Design review of the part built by this model. Coordinates are the model's own, in mm. A direction names the side the tool comes from. Give positions to 0.01 mm unless a question says otherwise; leave off trailing zeros. Write each loop counter-clockwise with the first axis right and the second up, starting at its lowest first coordinate (ties: lowest second). Pieces come first, ordered by that corner, then holes. Notation, with made-up numbers: (37.25, -15.75) -> (56.25, -15.75) arc R21 ccw to (56.25, 16.25) -> close; hole circle Ø8 at (-7.75, 14). An arc over 180 degrees is marked (long way). Answer as a JSON object with one key per item and string values.
Solid Edge part; units mm, degrees
sketch "Sketch1" plane through (0, 0, 0) normal (0, 0, 1) x (1, 0, 0)
  arc A0 (-42.2727, 39.6197) -> (-53.3598, 0) centre (-0.8768, 6.6744) ccw
  arc A1 (-53.3598, 0) -> (-25.9191, -47.548) centre (0.1673, -0.8009) ccw
  line L0 (-26.65, -48.8578) -> (-25.9191, -47.548)
  arc A2 (-54.8611, -0.0838) -> (-26.65, -48.8578) centre (0.1673, -0.8009) ccw
  arc A3 (-43.4475, 40.5523) -> (-54.8611, -0.0838) centre (-0.8768, 6.6744) ccw
  arc A4 (-9.2588, 61.3508) -> (-43.4475, 40.5523) centre (1.7356, 4.7791) ccw
  line L1 (-9.2588, 69.5332) -> (-9.2588, 61.3508)
  line L2 (5.3113, 69.5332) -> (-9.2588, 69.5332)
  line L3 (5.7406, 61.9223) -> (5.3113, 69.5332)
  arc A5 (43.4475, 40.5523) -> (5.7406, 61.9223) centre (-1.7356, 4.7791) ccw
  arc A6 (54.8611, -0.0838) -> (43.4475, 40.5523) centre (0.8768, 6.6744) ccw
  arc A7 (28.0706, -48.0371) -> (54.8611, -0.0838) centre (-0.1673, -0.8009) ccw
  line L4 (27.3009, -46.7496) -> (28.0706, -48.0371)
  arc A8 (53.3598, 0) -> (27.3009, -46.7496) centre (-0.1673, -0.8009) cw
  arc A9 (42.2727, 39.6197) -> (53.3598, 0) centre (0.8768, 6.6744) cw
  arc A10 (4.3138, 60.5824) -> (42.2727, 39.6197) centre (-1.7356, 4.7791) cw
  line L5 (3.8935, 68.0332) -> (4.3138, 60.5824)
  line L6 (-7.7588, 68.0332) -> (3.8935, 68.0332)
  line L7 (-7.7588, 68.0332) -> (-7.7588, 60.1005)
  arc A11 (-7.7588, 60.1005) -> (-42.2727, 39.6197) centre (1.7356, 4.7791) ccw
extrude "Protrusion1" add sketch "Sketch1" along normal blind 10
sketch "Sketch2" plane through (0, 10.3377, 10) normal (0, 0, 1) x (0, -1, 0)
  line L0 (8.4418, -53.9965) -> (8.4418, 54.1624)
  line L1 (8.4418, 54.1624) -> (10.3377, 53.3598)
  line L2 (10.3377, 53.3598) -> (10.3377, -53.3598)
  line L3 (10.3377, -53.3598) -> (8.4418, -53.9965)
extrude "ExtrudedProtrusion_2" add sketch "Sketch2" against normal blind 2
sketch "Sketch3" plane through (0, 10.3377, 10) normal (0, 0, 1) x (0, -1, 0)
  line L0 (58.3748, 28.0706) -> (10.3377, 0)
  line L1 (10.3377, 0) -> (10.3377, 2)
  line L2 (10.3377, 2) -> (56.6184, 28.0706)
  line L3 (56.6184, 28.0706) -> (58.3748, 28.0706)
extrude "ExtrudedProtrusion_3" add sketch "Sketch3" against normal blind 2
sketch "Sketch4" plane through (0, 10.3377, 10) normal (0, 0, 1) x (0, -1, 0)
  line L0 (10.3377, -2) -> (56.6184, -28.0706)
  line L1 (56.6184, -28.0706) -> (58.3748, -28.0706)
  line L2 (58.3748, -28.0706) -> (10.3377, 0)
extrude "ExtrudedProtrusion_4" add sketch "Sketch4" against normal blind 2 material side at (-14.9917, -23.1649, 10)
(1) For line 1 along Y through (x, z) = (-30.5, 8.75); line 2 along Y through (x, z) = (46, 9.5); line 3 along Y through (x, z) = (-28.5, 1.75), list the stretches that pass through material, from the lowest coordinate up.
Here are the results:
{"line 1": "y = -46.5 to -44.68, 0 to 1.9, 50.73 to 52.55", "line 2": "y = -30.75 to -27.9, 0 to 1.9, 34.3 to 37.07", "line 3": "y = -47.78 to -46.01, 52.07 to 53.84"}
(2) We need section A-A, the plane y = 56. State the section outline as (x, z) points.
Here are the results:
{"outline": "(-24.68, 0) -> (-21.22, 0) -> (-21.22, 10) -> (-24.68, 10) -> close; (21.22, 0) -> (24.68, 0) -> (24.68, 10) -> (21.22, 10) -> close"}
(3) Clearance check with flat-ended pins moving along their axes: pin 1 (6 mm diameter, centred on x = -21, z = 6, fed in from +Y); pin 2 (14.5 mm diameter, centred on x = -17, y = -21, fed in from -Z); pin 3 (2 mm diameter, centred on y = 56, z = 3.5, fed in from +X). State where each tip first meets the part, or that it passes through.
Here are the results:
{"pin 1": "stops at y = 58.92", "pin 2": "stops at z = 8", "pin 3": "stops at x = 26.53"}
(4) The part is to be moulded in two halves that separate along Y. For faces 1 (the flat face through (-14.853, -22.816, 9.014)), 2 (the cylindrical face through (-28.46, 53.865, 4.93)), 3 (the flat face through (24.8, 54.5, 0)), 4 (the flat face through (14.853, -22.816, 9.014)), say which applies: +Y half, -Y half, draft (parallel to the pull), parting line (faces both ways), or undercut.
Here are the results:
{"face 1": "undercut", "face 2": "+Y half", "face 3": "draft", "face 4": "undercut"}
(5) We need section D-D, the plane z = 4.5. State the section outline as (x, y) points, then the cut area to 3 significant figures.
Here are the results:
{"outline": "(-54.86, -0.08) arc R55.03 ccw to (-26.65, -48.86) -> (-25.92, -47.55) arc R53.53 cw to (-53.36, 0) arc R52.91 cw to (-42.27, 39.62) arc R56.13 cw to (-7.76, 60.1) -> (-7.76, 68.03) -> (3.89, 68.03) -> (4.31, 60.58) arc R56.13 cw to (42.27, 39.62) arc R52.91 cw to (53.36, 0) arc R53.53 cw to (27.3, -46.75) -> (28.07, -48.04) arc R55.03 ccw to (54.86, -0.08) arc R54.41 ccw to (43.45, 40.55) arc R57.63 ccw to (5.74, 61.92) -> (5.31, 69.53) -> (-9.26, 69.53) -> (-9.26, 61.35) arc R57.63 ccw to (-43.45, 40.55) arc R54.41 ccw to start", "area": "472 mm²"}
(6) For faces 5 (the flat face through (-4, -6, 8)), 6 (the flat face through (-2, 69.533, 5)), 7 (the flat face through (4.1, 64.4, 4.9)), 8 (the flat face through (-9.259, 65, 5)), list the 3-axis set-ups (+Z, -Z, +X, -X, +Y, -Y) from which the entire face can be reached by the end or side of a thin tool; tool diameter is ignored.
Here are the results:
{"face 5": "-Z", "face 6": "+Z, -Z, +X, -X, +Y", "face 7": "+Z, -Z", "face 8": "+Z, -Z, -X, +Y"}
(7) We need section B-B, the plane x = -13. State the section outline as (y, z) points, then the cut area to 3 significant figures.
Here are the results:
{"outline": "(-22.25, 8) -> (-19.53, 8) -> (-19.53, 10) -> (-22.25, 10) -> close; (0, 8) -> (1.9, 8) -> (1.9, 10) -> (0, 10) -> close; (58.94, 0) -> (60.49, 0) -> (60.49, 10) -> (58.94, 10) -> close", "area": "24.8 mm²"}
(8) We need section C-C, the plane y = -8.5. State the section outline as (x, z) points.
Here are the results:
{"outline": "(-54.32, 0) -> (-52.81, 0) -> (-52.81, 10) -> (-54.32, 10) -> close; (-6.79, 8) -> (-4.97, 8) -> (-4.97, 10) -> (-6.79, 10) -> close; (4.97, 8) -> (6.79, 8) -> (6.79, 10) -> (4.97, 10) -> close; (52.81, 0) -> (54.32, 0) -> (54.32, 10) -> (52.81, 10) -> close"}
